from build123d import *

# Parameters (mm, degrees)
F0_R     = 25
F1_DEPTH = 10
F2_R     = 60
F3_DEPTH = 10
F4_R     = 5
F5_DEPTH = 20.001
F6_R     = 17.6235
F7_DEPTH = 50


with BuildPart() as f1:
    # F0 (on Front) → F1 (new body)
    with BuildSketch(Plane.XZ):
        Circle(F0_R)
    extrude(amount=-F1_DEPTH)

    # F2 (on Front) → F3 (join)
    with BuildSketch(Plane.XZ):
        Circle(F2_R)
    extrude(amount=F3_DEPTH)

    # F4 (on face) → F5 (cut, through all)
    with BuildSketch(Plane.XZ.offset(10)):
        with Locations((0, 40)):
            Circle(F4_R)
        with Locations((-38.042261, 12.36068)):
            Circle(F4_R)
        with Locations((-23.51141, -32.36068)):
            Circle(F4_R)
        with Locations((23.51141, -32.36068)):
            Circle(F4_R)
        with Locations((38.042261, 12.36068)):
            Circle(F4_R)
    extrude(amount=-F5_DEPTH, mode=Mode.SUBTRACT)

    # F6 (on face) → F7 (cut)
    with BuildSketch(Plane.XZ.offset(10)):
        Circle(F6_R)
    extrude(amount=-F7_DEPTH, mode=Mode.SUBTRACT)


solid = f1.part
Read the model definition and answer for the solid it produces. Units are mm, in the model's axes. Give positions to 0.01 mm unless a question says otherwise; leave off trailing zeros. Write each loop counter-clockwise with the first axis right and the second up, starting at its lowest first coordinate (ties: lowest second). Pieces come first, ordered by that corner, then holes. Notation, with made-up numbers: M 22.5,7 L 79.5,7 A16 cw 79.5,24 Z; hole C -27.5,71.25 d7. An arc over 180 degrees is marked long. One line per item, written item: value. Start each with the question number.
(1) Find section B-B (x = 0). Determine the outline of the cut face in (y, z).
(2) Find section A-A (z = 0). Determine the outline of the cut face in (x, y).
(3) Determine the mould class of faces 1 (the cylindrical face through (16.81, -0.14, 5.29)), 2 (the flat face through (-1, 0, -26)), 3 (the cylindrical face through (23.846, 4.93, 7.509)) for opening direction X: pulls with the +X half, pulls with the -X half, needs draft (parallel to the pull), parting line crosses it, or undercut.
(4) Find the intervals of material crossed by line 1 (Z direction, x = -2.5, y = -2.5); line 2 (Z direction, x = -1, y = -4.25); line 3 (X direction, y = -1.25, z = 12.5), in increasing order.
(5) Find section D-D (y = 8.5). Determine the outline of the cut face in (x, z).
(6) Find section C-C (x = -38.5). Determine the outline of the cut face in (y, z).
(7) Flat-ended cylindrical pins translate along their axes: pin 1 Ø3 at (x, y) = (18.5, -2.5) entering from +Z; pin 2 Ø5 at (y, z) = (3, 11) entering from -X; pin 3 Ø12 at (x, y) = (-27, -0.5) entering from -Z (3 decimals). Find the tip coordinate at first contact, or state that the pin passes through.
Results below:
1. outline: M -10,-60 L 0,-60 L 0,-25 L 10,-25 L 10,-17.62 L -10,-17.62 Z; M -10,17.62 L 10,17.62 L 10,25 L 0,25 L 0,35 L -10,35 Z; M -10,45 L 0,45 L 0,60 L -10,60 Z
2. outline: M -60,-10 L -17.62,-10 L -17.62,10 L -25,10 L -25,0 L -60,0 Z; M 17.62,-10 L 60,-10 L 60,0 L 25,0 L 25,10 L 17.62,10 Z
3. face 1: undercut
3. face 2: needs draft
3. face 3: parting line crosses it
4. line 1: z = -59.95 to -17.45, 17.45 to 35.67, 44.33 to 59.95
4. line 2: z = -59.99 to -17.6, 17.6 to 35.1, 44.9 to 59.99
4. line 3: x = -58.68 to -43.04, -33.04 to -12.42, 12.42 to 33.04, 43.04 to 58.68
5. outline: C 0,0 d50; hole C 0,0 d35.25
6. outline: M -10,-46.02 L 0,-46.02 L 0,7.38 L -10,7.38 Z; M -10,17.34 L 0,17.34 L 0,46.02 L -10,46.02 Z
7. pin 1: stops at z = 57.54
7. pin 2: stops at x = -23.51
7. pin 3: stops at z = -56.205
